Check sheet for the modelled part. Datum: model origin and axes. Units: mm. Face numbers are marked on the shaded views. A direction names the side the tool comes from. Give positions to 0.01 mm unless a question says otherwise; leave off trailing zeros. Write each loop counter-clockwise with the first axis right and the second up, starting at its lowest first coordinate (ties: lowest second). Pieces come first, ordered by that corner, then holes.
from build123d import *

# Parameters (mm, degrees)
SKETCH1_W           = 40.2
SKETCH1_H           = 250
BOSS_EXTRUDE1_DEPTH = 10
SKETCH4_W           = 40.2
SKETCH4_H           = 247
CUT_EXTRUDE1_DEPTH  = 4.8
SKETCH3_W           = 29
SKETCH3_H           = 28.7
CUT_EXTRUDE2_DEPTH  = 11
SKETCH2_R           = 1.35
CUT_EXTRUDE3_DEPTH  = 11
SKETCH6_R           = 1.35
CUT_EXTRUDE4_DEPTH  = 251


with BuildPart() as part:
    # Sketch1 → Boss-Extrude1 (new body)
    with BuildSketch(Plane.XY):
        Rectangle(SKETCH1_W, SKETCH1_H)
    extrude(amount=BOSS_EXTRUDE1_DEPTH)

    # Sketch4 → Cut-Extrude1 (cut)
    with BuildSketch(Plane.XY.offset(10)):
        with Locations((0, -1.5)):
            Rectangle(SKETCH4_W, SKETCH4_H)
    extrude(amount=-CUT_EXTRUDE1_DEPTH, mode=Mode.SUBTRACT)

    # Sketch3 → Cut-Extrude2 (cut, through all)
    with BuildSketch(Plane.XY.offset(10)):
        with Locations((0, -110.65)):
            Rectangle(SKETCH3_W, SKETCH3_H)
    extrude(amount=-CUT_EXTRUDE2_DEPTH, mode=Mode.SUBTRACT)

    # Sketch2 → Cut-Extrude3 (cut, through all)
    with BuildSketch(Plane.XY.offset(10)):
        with Locations((17.3, -120.8)):
            Circle(SKETCH2_R)
        with Locations((11, -93.5)):
            Circle(SKETCH2_R)
        with Locations((-17.3, -120.8)):
            Circle(SKETCH2_R)
        with Locations((-11, -93.5)):
            Circle(SKETCH2_R)
    extrude(amount=-CUT_EXTRUDE3_DEPTH, mode=Mode.SUBTRACT)

    # Sketch6 → Cut-Extrude4 (cut, through all)
    with BuildSketch(Plane(origin=(0, 125, 0), x_dir=(-1, 0, 0), z_dir=(0, 1, 0))):
        with Locations((-17, 7.2)):
            Circle(SKETCH6_R)
        with Locations((17, 7.2)):
            Circle(SKETCH6_R)
        with Locations((0, 7.2)):
            Circle(SKETCH6_R)
    extrude(amount=-CUT_EXTRUDE4_DEPTH, mode=Mode.SUBTRACT)


solid = part.part
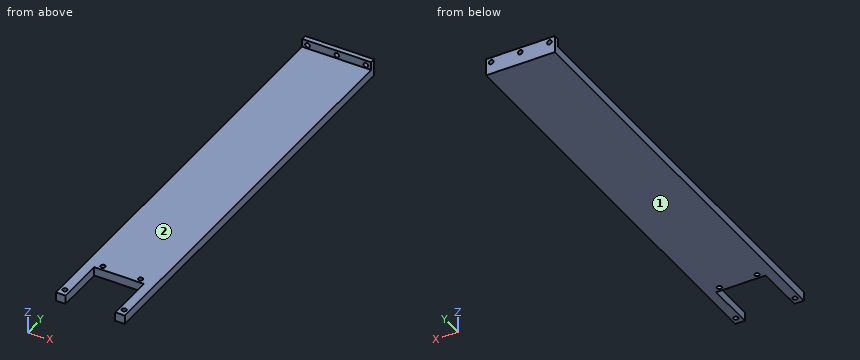
1) Scan lines: L1, parallel to X at y = -120.8, z = 3.2; L2, parallel to X at y = -93.5, z = 3.45; L3, parallel to Y at x = 17.3, z = 1.8. Record each from-to range of solid material in increasing order.
2) Sectioned sample at A-A on z = 1.75. Record the boundary of the cut face in (x, y), then the cut area to 3 significant figures.
3) Access from +Z, -Z, +X, -X, +Y, -Y to the whole of each face (thin tool, end or side, straight path). Record for the marked faces 1 and 2.
4) Sectioned sample at C-C on y = -43. Record the boundary of the cut face in (x, z), then the cut area to 3 significant figures.
5) Sectioned sample at B-B on x = -3.5. Record the boundary of the cut face in (y, z), then the cut area to 3 significant figures.
6) Gauge pin test, flat ends, axial feed: pin 1 (20 mm diameter, centred on x = 7.5, y = -19, fed in from +Z); pin 2 (3.5 mm diameter, centred on x = -17, z = 7.2, fed in from +Y); pin 3 (4 mm diameter, centred on x = 10, z = 3.5, fed in from -Y); pin 4 (1.6 mm diameter, centred on x = 11, y = -93.5, fed in from +Z). Record the tip position at first contact, or that the pin passes through.
Answers below:
1. L1: x = -20.1 to -18.65, -15.95 to -14.5, 14.5 to 15.95, 18.65 to 20.1
1. L2: x = -20.1 to -12.35, -9.65 to 9.65, 12.35 to 20.1
1. L3: y = -125 to -122.15, -119.45 to 125
2. outline: (-20.1, -125) - (-14.5, -125) - (-14.5, -96.3) - (14.5, -96.3) - (14.5, -125) - (20.1, -125) - (20.1, 125) - (-20.1, 125) - close; hole circle Ø2.7 at (-17.3, -120.8); hole circle Ø2.7 at (-11, -93.5); hole circle Ø2.7 at (11, -93.5); hole circle Ø2.7 at (17.3, -120.8)
2. area: 9,190 mm2
3. face 1: -Z, +X, -X, +Y, -Y
3. face 2: +Z, +X, -X, -Y
4. outline: (-20.1, 0) - (20.1, 0) - (20.1, 5.2) - (-20.1, 5.2) - close
4. area: 209 mm2
5. outline: (-96.3, 0) - (125, 0) - (125, 10) - (122, 10) - (122, 5.2) - (-96.3, 5.2) - close
5. area: 1,170 mm2
6. pin 1: stops at z = 5.2
6. pin 2: stops at y = 125
6. pin 3: stops at y = -96.3
6. pin 4: passes through
